Source: three-view drawing plus pictorial views. Frame: mm from the lowest corner of the part. Give positions to 0.01 mm unless a question says otherwise; leave off trailing zeros. Order: outer loops, then holes, each group sorted by start corner. A loop starts at its lowest first (then second) coordinate and runs counter-clockwise, first axis right, second up. Notation, with made-up numbers: (22.5, 56.5) - (52.5, 56.5) arc R21 ccw to (52.5, 70.5) - close; hole circle Ø4 at (89.25, -23.75). An arc over 180 degrees is marked (long way). Answer in a Markdown table with one row per item. Add a question column.
1. Ray query, line 1 (Z direction, x = 2.6, y = 10); line 2 (Y direction, x = 1.1, z = 1.7). Return the intervals inside material, ascending. Write a range as [from, to].
2. Section query A-A on y = 10.25. Return loops of the section in (x, z).
3. Mould query, pull axis Z, two halves, no side actions, for the marked faces 1, 2 and 3. Classes: released by +Z, released by -Z, zero draft, split by the parting line, or undercut.
4. Contact query for flat-ended pins moving along their axis: pin 1 (0.8 mm diameter, centred on x = 3, z = 3, fed in from +Y); pin 2 (2 mm diameter, centred on y = 7.5, z = 4, fed in from +X) (1 decimal); pin 3 (1 mm diameter, centred on x = 0.5, y = 8, fed in from +Z); pin 4 (0.6 mm diameter, centred on x = 3, y = 14, fed in from -Z). Output: stop coordinate, or through.
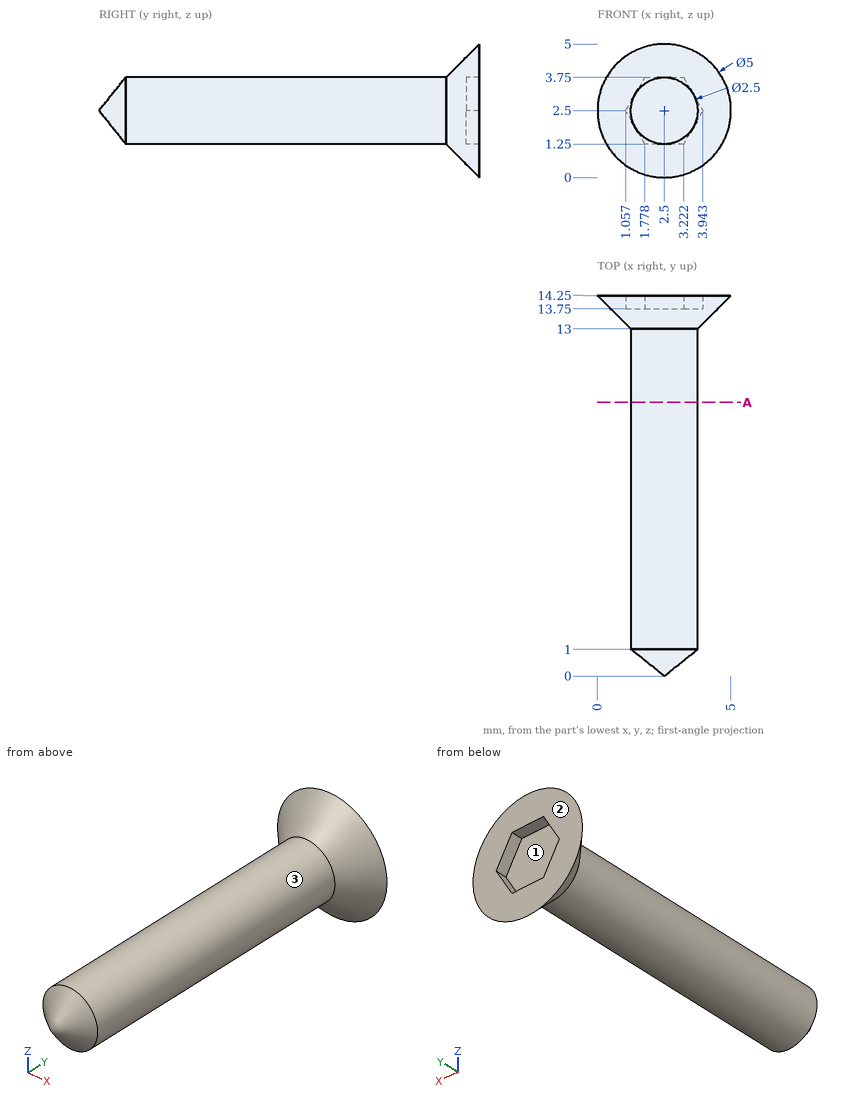
Answer:
| question | item | result |
|---|---|---|
| 1 | line 1 | z = [1.25, 3.75] |
| 1 | line 2 | y = [13.36, 14.25] |
| 2 | outline | circle Ø2.5 at (2.5, 2.5) |
| 3 | face 1 | undercut |
| 3 | face 2 | zero draft |
| 3 | face 3 | split by the parting line |
| 4 | pin 1 | stops at y = 13.75 |
| 4 | pin 2 | stops at x = 3.6 |
| 4 | pin 3 | passes through |
| 4 | pin 4 | stops at z = 0.02 |
